Source: CAD feature listing. Evaluate the final solid. Frame: model axes, mm. Face numbers are marked on the shaded views. A direction names the side the tool comes from. Round coordinates to 2 decimals unless told otherwise and drop trailing zeros. Loops run counter-clockwise (first coordinate to the right, second up) from the corner with the lowest first, then second, coordinate; pieces in that order, holes last. Notation, with made-up numbers: (-4, -25) - (3, -25) arc R20 ccw to (3, -6) - close; hole circle Ø7 at (81.5, 68). An arc over 180 degrees is marked (long way). Write item = value, one per line. Start each with the question number.
from build123d import *

# Parameters (mm, degrees)
EXTRUDE_1_DEPTH          = 2.9
SKETCH_2_R               = 1.55
SKETCH_2_W               = 8.5
SKETCH_2_H               = 4.425
CUT_EXTRUDE_1_DEPTH      = 10
FILLET_1_R               = 2
HOLE_WIZARD_1_AT_2_COUNT = 2
HOLE_WIZARD_1_AT_2_PITCH = 14


with BuildPart() as part:
    # 草图1 → 凸台-拉伸1 (new body)
    with BuildSketch(Plane(origin=(0, 0, 0), x_dir=(0, 0, -1), z_dir=(1, 0, 0))):
        with BuildLine():
            Line((-12, 15.425), (-12, 12.425))
            ThreePointArc((-12, 12.425), (-13.05, 11.375), (-14.1, 12.425))
            Line((-14.1, 12.425), (-18, 12.425))
            Line((-18, 12.425), (-18, -12.425))
            Line((-18, -12.425), (-14.1, -12.425))
            ThreePointArc((-14.1, -12.425), (-13.05, -11.375), (-12, -12.425))
            Line((-12, -12.425), (-12, -15.425))
            Line((-12, -15.425), (-4, -15.425))
            Line((-4, -15.425), (-4, -12.425))
            ThreePointArc((-4, -12.425), (-2.95, -11.375), (-1.9, -12.425))
            Line((-1.9, -12.425), (1.9, -12.425))
            ThreePointArc((1.9, -12.425), (2.95, -11.375), (4, -12.425))
            Line((4, -12.425), (4, -15.425))
            Line((4, -15.425), (12, -15.425))
            Line((12, -15.425), (12, -12.425))
            ThreePointArc((12, -12.425), (13.05, -11.375), (14.1, -12.425))
            Line((14.1, -12.425), (18, -12.425))
            Line((18, -12.425), (18, 12.425))
            Line((18, 12.425), (14.1, 12.425))
            ThreePointArc((14.1, 12.425), (13.05, 11.375), (12, 12.425))
            Line((12, 12.425), (12, 15.425))
            Line((12, 15.425), (4, 15.425))
            Line((4, 15.425), (4, 12.425))
            ThreePointArc((4, 12.425), (2.95, 11.375), (1.9, 12.425))
            Line((1.9, 12.425), (-1.9, 12.425))
            ThreePointArc((-1.9, 12.425), (-2.95, 11.375), (-4, 12.425))
            Line((-4, 12.425), (-4, 15.425))
            Line((-4, 15.425), (-12, 15.425))
        make_face()
    extrude(amount=EXTRUDE_1_DEPTH)

    # 草图2 → 切除-拉伸1 (cut)
    with BuildSketch(Plane.ZY):
        with Locations((-15, 7.5)):
            Circle(SKETCH_2_R)
        with Locations(Location((-15, -7.5, 0), (0, 0, 180))):
            Circle(SKETCH_2_R)
        with Locations((15, 0)):
            Circle(SKETCH_2_R)
        with Locations((-15, 0)):
            Circle(SKETCH_2_R)
        with Locations((15, -7.5)):
            Circle(SKETCH_2_R)
        with Locations(Location((15, 7.5, 0), (0, 0, 180))):
            Circle(SKETCH_2_R)
        with Locations((-7, 0)):
            Circle(SKETCH_2_R)
        with Locations((7, 0)):
            Circle(SKETCH_2_R)
        with Locations((-6.75, 5.7125)):
            Rectangle(SKETCH_2_W, SKETCH_2_H)
        with Locations((-6.75, -5.7125)):
            Rectangle(SKETCH_2_W, SKETCH_2_H)
        with Locations((6.75, -5.7125)):
            Rectangle(SKETCH_2_W, SKETCH_2_H)
        with Locations((6.75, 5.7125)):
            Rectangle(SKETCH_2_W, SKETCH_2_H)
    extrude(amount=-CUT_EXTRUDE_1_DEPTH, mode=Mode.SUBTRACT)

    # 圆角1
    fillet_1_edges = [part.edges().sort_by_distance(p)[0] for p in [
        (1.45, -3.5, -2.5),
        (1.45, -7.925, -2.5),
        (1.45, -7.925, -11),
        (1.45, -3.5, -11),
        (1.45, 3.5, -11),
        (1.45, 7.925, -11),
        (1.45, 7.925, -2.5),
        (1.45, 3.5, -2.5),
        (1.45, 7.925, 11),
        (1.45, 3.5, 11),
        (1.45, 3.5, 2.5),
        (1.45, 7.925, 2.5),
        (1.45, -7.925, 11),
        (1.45, -7.925, 2.5),
        (1.45, -3.5, 2.5),
        (1.45, -3.5, 11),
    ]]
    fillet(fillet_1_edges, radius=FILLET_1_R)

    # 草图3 → 打孔尺寸(%根据十字)槽沉头木螺钉的类型1 (revolve, cut)
    with BuildSketch(Plane(origin=(2.9, 0, 7), x_dir=(0, 0, -1), z_dir=(0, 1, 0))):
        Polygon((0, 0), (0, 2.9), (1.55, 2.9), (1.55, 1.75), (3.3, 0), align=None)
    hole_wizard_1 = revolve(axis=Axis((9.25, 0, 7), (-1, 0, 0)), mode=Mode.SUBTRACT)

    # 打孔尺寸(%根据十字)槽沉头木螺钉的类型1 at 2: 打孔尺寸(%根据十字)槽沉头木螺钉的类型1 ×2
    with Locations(*[(0, 0, -i * HOLE_WIZARD_1_AT_2_PITCH) for i in range(1, HOLE_WIZARD_1_AT_2_COUNT)]):
        add(hole_wizard_1, mode=Mode.SUBTRACT)


solid = part.part
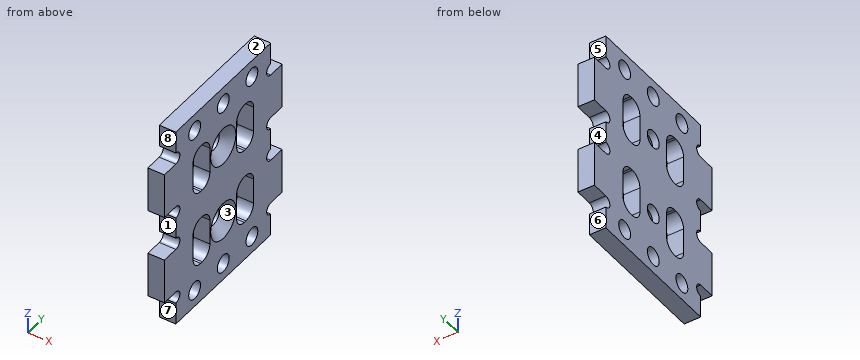
(1) Cut plane B-B (y = 7.5). Output: boundary loops of the cut face in (x, z), and give its area (3 significant figures).
(2) Material intervals for line 1 along Y through (x, z) = (1.8, -15) (3 decimals); line 2 along Y through (x, z) = (0.35, -6) (3 decimals); line 3 along Y through (x, z) = (2.1, 3), sorted ascending. Write a range as from..to.
(3) Cut plane A-A (z = -15). Output: boundary loops of the cut face in (x, y) (3 decimals), and give its area (3 significant figures).
(4) Pin query (flat end, axial travel): P1, Ø1.5, axis at x = 1.5, z = -0.5, coming from the -Y side (3 decimals). Return the tip coordinate at first contact, or that it passes through.
(5) Access query for the marked faces 4, 5, 6, 7 and 8. Directions: +Z, -Z, +X, -X, +Y, -Y. A direction counts if a zero-diameter tool reaches every point of the face in a straight line with its end or side. Return the directions, or none.
(6) Mould query, pull axis Y, two halves, no side actions, for the marked faces 1, 2 and 3. Classes: +Y half, -Y half, draft (parallel to the pull), parting line (faces both ways), or undercut.
(7) Cut plane D-D (x = 2.5). State how many separate pieces and enclosed holes the cut face has, and give its area (3 significant figures).
(8) Cut plane C-C (z = -2.95). Output: boundary loops of the cut face in (x, y) (3 decimals).
Solution:
q1.outline = (0, -18) - (2.9, -18) - (2.9, -16.55) - (0, -16.55) - close; (0, -13.45) - (2.9, -13.45) - (2.9, -10.23) - (0, -10.23) - close; (0, -3.27) - (2.9, -3.27) - (2.9, 3.27) - (0, 3.27) - close; (0, 10.23) - (2.9, 10.23) - (2.9, 13.45) - (0, 13.45) - close; (0, 16.55) - (2.9, 16.55) - (2.9, 18) - (0, 18) - close
q1.area = 46.0 mm^2
q2.line_1 = -12.425..-9.05, -5.95..-1.55, 1.55..5.95, 9.05..12.425
q2.line_2 = -15.425..-7.925, -3.5..-1.184, 1.184..3.5, 7.925..15.425
q2.line_3 = -11.38..-7.25, -4.18..4.18, 7.25..11.38
q3.outline = (0, -12.425) - (2.9, -12.425) - (2.9, -9.05) - (0, -9.05) - close; (0, -5.95) - (2.9, -5.95) - (2.9, -1.55) - (0, -1.55) - close; (0, 1.55) - (2.9, 1.55) - (2.9, 5.95) - (0, 5.95) - close; (0, 9.05) - (2.9, 9.05) - (2.9, 12.425) - (0, 12.425) - close
q3.area = 45.1 mm^2
q4.P1 = -12.425
q5.face_4 = +X, -X, +Y
q5.face_5 = +Z, +X, -X, +Y
q5.face_6 = -Z, +X, -X, +Y
q5.face_7 = -Z, +X, -X, -Y
q5.face_8 = +Z, +X, -X, -Y
q6.face_1 = -Y half
q6.face_2 = draft
q6.face_3 = undercut
q7.separate_pieces = 1
q7.enclosed_holes = 12
q7.area = 742 mm^2
q8.outline = (0, -11.375) - (2.9, -11.375) - (2.9, -7.189) - (0, -7.189) - close; (0, -4.236) - (2.9, -4.236) - (2.9, 4.236) - (0, 4.236) - close; (0, 7.189) - (2.9, 7.189) - (2.9, 11.375) - (0, 11.375) - close
